Work out the finished part from the listing and answer in its coordinate system (mm). A direction names the side the tool comes from. Give positions to 0.01 mm unless a question says otherwise; leave off trailing zeros. Write each loop counter-clockwise with the first axis right and the second up, starting at its lowest first coordinate (ties: lowest second). Pieces come first, ordered by that corner, then holes.
1) Straight lines are drawn through the part: probe 1 along X at (y, z) = (0.45, -15); probe 2 along Y at (x, z) = (39.5, -28.75); probe 3 along X at (y, z) = (12, -6). For each, find the intervals that lie inside material, in ascending order.
2) Find section A-A (z = -28.75). Determine the outline of the cut face in (x, y) (3 decimals), plus the area to 3 significant figures.
3) Given pin 1 Ø0.8 at (y, z) = (16.5, -29) entering from +X; pin 2 Ø5 at (x, z) = (29.5, -42.5) entering from +Y; pin 3 Ø2.5 at (x, z) = (7, -15) entering from +Y; pin 4 Ø1.4 at (x, y) = (22.75, 11.5) entering from +Z, each flat-ended and moving along its own axis, determine where each tip first touches the part or whether it passes through.
4) Find section D-D (x = 22.75). Determine the outline of the cut face in (y, z).
5) Find section B-B (x = 33). Determine the outline of the cut face in (y, z).
6) Find section C-C (z = -11.5). Determine the outline of the cut face in (x, y).
7) A tool of negligible diameter and unlimited length cuts with its end or side. For faces 1 (the face through (38.53, 15.71, -29.44)), 2 (the face through (15.869, 9.675, -6.958)), 3 (the face through (8.352, 3.014, -43.974)), from which of +Z, -Z, +X, -X, +Y, -Y can it reach the whole face along a straight path? Write none if from no direction.
8) Determine the mould class of faces 4 (the face through (40.5, 14.3, -27.3)), 5 (the face through (18, 7, -8)), 6 (the face through (22.2, 12.01, -5.97)) for opening direction Z: pulls with the +Z half, pulls with the -Z half, needs draft (parallel to the pull), parting line crosses it, or undercut.
```python
from build123d import *

# Parameters (mm, degrees)
EXTRUDE_1_DEPTH     = 19
SHELL_START         = 4
SHELL_2_DEPTH       = 15
SKETCH_2_R          = 3
CUT_EXTRUDE_1_DEPTH = 15
SKETCH_3_R          = 6
CUT_EXTRUDE_2_DEPTH = 4
SKETCH_4_R          = 3
CUT_EXTRUDE_3_DEPTH = 18
SKETCH_5_R          = 6
CUT_EXTRUDE_4_DEPTH = 4
SKETCH_8_R          = 0.75
CUT_EXTRUDE_5_DEPTH = 4
SKETCH_9_R          = 0.75
CUT_EXTRUDE_6_DEPTH = 4
EXTRUDE_4_DEPTH     = 1
EXTRUDE_5_DEPTH     = 1
SKETCH_13_R         = 2
CUT_EXTRUDE_7_DEPTH = 2
SKETCH_14_R         = 1.5
CUT_EXTRUDE_8_DEPTH = 9


# Read off the part's stored shape, not the designer's step: 抽壳2
with BuildPart() as part:
    # 草图1 → 凸台-拉伸1 (new body)
    with BuildSketch(Plane(origin=(0, 0, 0), x_dir=(1, 0, 0), z_dir=(0, 1, 0))):
        with BuildLine():
            Line((5, 0), (44.5, 0))
            Line((44.5, 0), (44.5, 49.5))
            Line((44.5, 49.5), (5, 49.5))
            ThreePointArc((5, 49.5), (1.464466094, 48.035533906), (0, 44.5))
            Line((0, 44.5), (0, 5))
            ThreePointArc((0, 5), (1.464466094, 1.464466094), (5, 0))
        make_face()
    extrude(amount=EXTRUDE_1_DEPTH)

    # 抽壳2 outline → 抽壳2 (cut)
    with BuildSketch(Plane(origin=(0, 0, 0), x_dir=(1, 0, 0), z_dir=(0, 1, 0)).offset(SHELL_START)):
        with BuildLine():
            ThreePointArc((5, 47.5), (2.878679656, 46.621320344), (2, 44.5))
            Line((2, 44.5), (2, 10))
            Line((2, 10), (34.5, 10))
            Line((34.5, 10), (34.5, 47.5))
            Line((34.5, 47.5), (5, 47.5))
        make_face()
    extrude(amount=SHELL_2_DEPTH, mode=Mode.SUBTRACT)

    # 草图2 → 切除-拉伸1 (cut)
    with BuildSketch(Plane.XY):
        with Locations((18.25, 11.5)):
            Circle(SKETCH_2_R)
    extrude(amount=-CUT_EXTRUDE_1_DEPTH, mode=Mode.SUBTRACT)

    # 草图3 → 切除-拉伸2 (cut)
    with BuildSketch(Plane.XY):
        with Locations((18.25, 11.5)):
            Circle(SKETCH_3_R)
    extrude(amount=-CUT_EXTRUDE_2_DEPTH, mode=Mode.SUBTRACT)

    # 草图4 → 切除-拉伸3 (cut)
    with BuildSketch(Plane(origin=(44.5, 0, 0), x_dir=(0, 0, -1), z_dir=(1, 0, 0))):
        with Locations((28.75, 11.5)):
            Circle(SKETCH_4_R)
    extrude(amount=-CUT_EXTRUDE_3_DEPTH, mode=Mode.SUBTRACT)

    # 草图5 → 切除-拉伸4 (cut)
    with BuildSketch(Plane(origin=(44.5, 0, 0), x_dir=(0, 0, -1), z_dir=(1, 0, 0))):
        with Locations((28.75, 11.5)):
            Circle(SKETCH_5_R)
    extrude(amount=-CUT_EXTRUDE_4_DEPTH, mode=Mode.SUBTRACT)

    # 草图8 → 切除-拉伸5 (cut)
    with BuildSketch(Plane(origin=(40.5, 0, 0), x_dir=(0, 0, -1), z_dir=(1, 0, 0))):
        with Locations((28.75, 16)):
            Circle(SKETCH_8_R)
        with Locations((33.25, 11.5)):
            Circle(SKETCH_8_R)
        with Locations((24.25, 11.5)):
            Circle(SKETCH_8_R)
        with Locations((28.75, 7)):
            Circle(SKETCH_8_R)
    extrude(amount=-CUT_EXTRUDE_5_DEPTH, mode=Mode.SUBTRACT)

    # 草图9 → 切除-拉伸6 (cut)
    with BuildSketch(Plane.XY.offset(-4)):
        with Locations((18.25, 16)):
            Circle(SKETCH_9_R)
        with Locations((22.75, 11.5)):
            Circle(SKETCH_9_R)
        with Locations((18.25, 7)):
            Circle(SKETCH_9_R)
        with Locations((13.75, 11.5)):
            Circle(SKETCH_9_R)
    extrude(amount=-CUT_EXTRUDE_6_DEPTH, mode=Mode.SUBTRACT)

    # 草图10 → 凸台-拉伸4 (add)
    with BuildSketch(Plane.XY.offset(-47.5)):
        with BuildLine():
            Line((9.594076089, 19), (26.905923911, 19))
            ThreePointArc((26.905923911, 19), (18.25, 4.0075), (9.594076089, 19))
        make_face()
    extrude(amount=EXTRUDE_4_DEPTH)

    # 草图11 → 凸台-拉伸5 (add)
    with BuildSketch(Plane(origin=(2, 0, 0), x_dir=(0, 0, -1), z_dir=(1, 0, 0))):
        with BuildLine():
            Line((19.825313731, 19), (37.674686269, 19))
            ThreePointArc((37.674686269, 19), (28.75, 4.505), (19.825313731, 19))
        make_face()
    extrude(amount=EXTRUDE_5_DEPTH)

    # 草图13 → 切除-拉伸7 (cut)
    with BuildSketch(Plane(origin=(0, 4, 0), x_dir=(1, 0, 0), z_dir=(0, 1, 0))):
        with Locations(Location((7, 15, 0), (0, 0, 270))):
            Circle(SKETCH_13_R)
        with Locations(Location((7, 42.5, 0), (0, 0, 270))):
            Circle(SKETCH_13_R)
        with Locations(Location((29.5, 15, 0), (0, 0, 270))):
            Circle(SKETCH_13_R)
        with Locations(Location((29.5, 42.5, 0), (0, 0, 270))):
            Circle(SKETCH_13_R)
    extrude(amount=-CUT_EXTRUDE_7_DEPTH, mode=Mode.SUBTRACT)

    # 草图14 → 切除-拉伸8 (cut)
    with BuildSketch(Plane(origin=(0, 4, 0), x_dir=(1, 0, 0), z_dir=(0, 1, 0))):
        with Locations(Location((7, 15, 0), (0, 0, 270))):
            Circle(SKETCH_14_R)
        with Locations(Location((7, 42.5, 0), (0, 0, 270))):
            Circle(SKETCH_14_R)
        with Locations(Location((29.5, 15, 0), (0, 0, 270))):
            Circle(SKETCH_14_R)
        with Locations(Location((29.5, 42.5, 0), (0, 0, 270))):
            Circle(SKETCH_14_R)
    extrude(amount=-CUT_EXTRUDE_8_DEPTH, mode=Mode.SUBTRACT)


solid = part.part
```
Results:
1. probe 1: x = 0 to 5.5, 8.5 to 28, 31 to 44.5
1. probe 2: y = 0 to 6.25, 7.75 to 8.5, 14.5 to 15.25, 16.75 to 19
1. probe 3: x = 0 to 13.19, 14.31 to 15.29, 21.21 to 22.19, 23.31 to 44.5
2. outline: (0, 0) - (44.5, 0) - (44.5, 5.5) - (40.5, 5.5) - (40.5, 6.25) - (36.5, 6.25) - (36.5, 7.75) - (40.5, 7.75) - (40.5, 8.5) - (34.5, 8.5) - (34.5, 4) - (2, 4) - (2, 4.505) - (3, 4.505) - (3, 19) - (0, 19) - close; (34.5, 14.5) - (40.5, 14.5) - (40.5, 15.25) - (36.5, 15.25) - (36.5, 16.75) - (40.5, 16.75) - (40.5, 17.5) - (44.5, 17.5) - (44.5, 19) - (34.5, 19) - close
2. area: 276 mm2
3. pin 1: stops at x = 40.5
3. pin 2: stops at y = 4
3. pin 3: passes through
3. pin 4: stops at z = -8
4. outline: (0, -49.5) - (19, -49.5) - (19, -46.5) - (5.08, -46.5) - (5.08, -47.5) - (4, -47.5) - (4, -10) - (19, -10) - (19, 0) - (15.47, 0) - (15.47, -4) - (12.25, -4) - (12.25, -8) - (10.75, -8) - (10.75, -4) - (7.53, -4) - (7.53, 0) - (0, 0) - close
5. outline: (0, -49.5) - (19, -49.5) - (19, -47.5) - (4, -47.5) - (4, -10) - (19, -10) - (19, 0) - (0, 0) - close
6. outline: (0, 0) - (44.5, 0) - (44.5, 19) - (34.5, 19) - (34.5, 4) - (2, 4) - (2, 19) - (0, 19) - close
7. face 1: +X
7. face 2: +Z
7. face 3: +Y
8. face 4: undercut
8. face 5: pulls with the +Z half
8. face 6: needs draft
